Model file for the job. Use its own axes, mm. A direction names the side the tool comes from. Round coordinates to 2 decimals unless told otherwise and drop trailing zeros. Order: outer loops, then holes, each group sorted by start corner. A loop starts at its lowest first (then second) coordinate and runs counter-clockwise, first axis right, second up. Notation, with made-up numbers: (55, 35.25) - (89, 35.25) arc R21 cw to (89, 60.25) - close; hole circle Ø6 at (-9.5, 73). An arc over 180 degrees is marked (long way). Write item = value, one per line. Start each with the question number.
Autodesk Inventor part; units mm, degrees
ref_plane "YZ Plane" through (0, 0, 0) normal (1, 0, 0) x (0, 1, 0)
ref_plane "XZ Plane" through (0, 0, 0) normal (0, 1, 0) x (-1, 0, 0)
ref_plane "XY Plane" through (0, 0, 0) normal (0, 0, 1) x (1, 0, 0)
sketch "Sketch1" plane through (0, 0, 0) normal (0, 0, 1) x (1, 0, 0)
  line L0 (-9.652, -11.176) -> (9.652, -11.176)
  arc A0 (-11.176, -9.652) -> (-9.652, -11.176) centre (-9.652, -9.652) ccw
  line L1 (-11.176, 9.652) -> (-11.176, -9.652)
  arc A1 (-9.652, 11.176) -> (-11.176, 9.652) centre (-9.652, 9.652) ccw
  line L2 (9.652, 11.176) -> (-9.652, 11.176)
  arc A2 (11.176, 9.652) -> (9.652, 11.176) centre (9.652, 9.652) ccw
  line L3 (11.176, -9.652) -> (11.176, 9.652)
  arc A3 (9.652, -11.176) -> (11.176, -9.652) centre (9.652, -9.652) ccw
  arc A4 (12.7, 6.731) -> (13.081, 6.35) centre (13.081, 6.731) ccw
  line L4 (12.7, 6.731) -> (12.7, 10.5918)
  arc A5 (12.7, 10.5918) -> (10.5918, 12.7) centre (10.5918, 10.5918) ccw
  line L5 (10.5918, 12.7) -> (-10.5918, 12.7)
  arc A6 (-10.5918, 12.7) -> (-12.7, 10.5918) centre (-10.5918, 10.5918) ccw
  line L6 (-12.7, 10.5918) -> (-12.7, 6.731)
  arc A7 (-13.081, 6.35) -> (-12.7, 6.731) centre (-13.081, 6.731) ccw
  line L7 (-13.081, 6.35) -> (-25.019, 6.35)
  arc A8 (-25.019, 6.35) -> (-25.4, 5.969) centre (-25.019, 5.969) ccw
  line L8 (-25.4, 5.969) -> (-25.4, 4.826)
  arc A9 (-25.4, 4.826) -> (-24.638, 4.064) centre (-24.638, 4.826) ccw
  line L9 (-24.638, 4.064) -> (-23.0632, 4.064)
  arc A10 (-23.0632, 4.064) -> (-22.6822, 4.445) centre (-23.0632, 4.445) ccw
  arc A11 (-22.3012, 4.826) -> (-22.6822, 4.445) centre (-22.3012, 4.445) ccw
  line L10 (-22.3012, 4.826) -> (-13.081, 4.826)
  arc A12 (-12.7, 4.445) -> (-13.081, 4.826) centre (-13.081, 4.445) ccw
  line L11 (-12.7, 4.445) -> (-12.7, -4.445)
  arc A13 (-13.081, -4.826) -> (-12.7, -4.445) centre (-13.081, -4.445) ccw
  line L12 (-13.081, -4.826) -> (-22.3012, -4.826)
  arc A14 (-22.6822, -4.445) -> (-22.3012, -4.826) centre (-22.3012, -4.445) ccw
  arc A15 (-22.6822, -4.445) -> (-23.0632, -4.064) centre (-23.0632, -4.445) ccw
  line L13 (-23.0632, -4.064) -> (-24.638, -4.064)
  arc A16 (-24.638, -4.064) -> (-25.4, -4.826) centre (-24.638, -4.826) ccw
  line L14 (-25.4, -4.826) -> (-25.4, -5.969)
  arc A17 (-25.4, -5.969) -> (-25.019, -6.35) centre (-25.019, -5.969) ccw
  line L15 (-25.019, -6.35) -> (-13.081, -6.35)
  arc A18 (-12.7, -6.731) -> (-13.081, -6.35) centre (-13.081, -6.731) ccw
  line L16 (-12.7, -6.731) -> (-12.7, -10.5918)
  arc A19 (-12.7, -10.5918) -> (-10.5918, -12.7) centre (-10.5918, -10.5918) ccw
  line L17 (-10.5918, -12.7) -> (10.5918, -12.7)
  arc A20 (10.5918, -12.7) -> (12.7, -10.5918) centre (10.5918, -10.5918) ccw
  line L18 (12.7, -10.5918) -> (12.7, -6.731)
  arc A21 (13.081, -6.35) -> (12.7, -6.731) centre (13.081, -6.731) ccw
  line L19 (13.081, -6.35) -> (25.019, -6.35)
  arc A22 (25.019, -6.35) -> (25.4, -5.969) centre (25.019, -5.969) ccw
  line L20 (25.4, -5.969) -> (25.4, -4.826)
  arc A23 (25.4, -4.826) -> (24.638, -4.064) centre (24.638, -4.826) ccw
  line L21 (24.638, -4.064) -> (23.0632, -4.064)
  arc A24 (23.0632, -4.064) -> (22.6822, -4.445) centre (23.0632, -4.445) ccw
  arc A25 (22.3012, -4.826) -> (22.6822, -4.445) centre (22.3012, -4.445) ccw
  line L22 (22.3012, -4.826) -> (13.081, -4.826)
  arc A26 (12.7, -4.445) -> (13.081, -4.826) centre (13.081, -4.445) ccw
  line L23 (12.7, -4.445) -> (12.7, 4.445)
  arc A27 (13.081, 4.826) -> (12.7, 4.445) centre (13.081, 4.445) ccw
  line L24 (13.081, 4.826) -> (22.3012, 4.826)
  arc A28 (22.6822, 4.445) -> (22.3012, 4.826) centre (22.3012, 4.445) ccw
  arc A29 (22.6822, 4.445) -> (23.0632, 4.064) centre (23.0632, 4.445) ccw
  line L25 (23.0632, 4.064) -> (24.638, 4.064)
  arc A30 (24.638, 4.064) -> (25.4, 4.826) centre (24.638, 4.826) ccw
  line L26 (25.4, 4.826) -> (25.4, 5.969)
  arc A31 (25.4, 5.969) -> (25.019, 6.35) centre (25.019, 5.969) ccw
  line L27 (25.019, 6.35) -> (13.081, 6.35)
  point P0 (0, 0)
extrude "Extrusion1" add sketch "Sketch1" against normal blind 304.8
properties part number "9035"
Item 1: Mould opens along X. For faces 1 (the face through (-11.176, 0, -150)), 2 (the face through (19, -6.35, -150)) say: +X half, -X half, draft (parallel to the pull), parting line (faces both ways), or undercut.
Item 2: Saw through at A-A, the plane x = -18. Give the cut face in (y, z).
Item 3: Drop flat-ended pins along their axis: pin 1 (3 mm diameter, centred on y = -9, z = -213.5, fed in from -X); pin 2 (10 mm diameter, centred on x = -19, z = -87.5, fed in from +Y); pin 3 (1.3 mm diameter, centred on x = 24, z = -118.5, fed in from -Y). Give the stop position or say it passes through.
Item 4: Probe L1, parallel to X at y = 7, z = -275; L2, parallel to Y at x = -18, z = -76.5. List the from-to ranges inside material, lowest first.
Item 5: Which spindle directions (+Z, -Z, +X, -X, +Y, -Y) get a long thin tool onto all of the face, cutting with end or side? Do faces 3 (the face through (0, -12.7, -150)), 4 (the face through (-18, 4.826, -150)), 5 (the face through (-19, -6.35, -150)), 6 (the face through (19, 6.35, -150)), 7 (the face through (-19, 6.35, -150)). Say none if no direction does.
Check sheet entries:
q1.face_1 = undercut
q1.face_2 = draft
q2.outline = (-6.35, -304.8) - (-4.83, -304.8) - (-4.83, 0) - (-6.35, 0) - close; (4.83, -304.8) - (6.35, -304.8) - (6.35, 0) - (4.83, 0) - close
q3.pin_1 = -12.7
q3.pin_2 = 6.35
q3.pin_3 = -6.35
q4.L1 = -12.7 to -11.18, 11.18 to 12.7
q4.L2 = -6.35 to -4.83, 4.83 to 6.35
q5.face_3 = +Z, -Z, +X, -X, -Y
q5.face_4 = +Z, -Z
q5.face_5 = +Z, -Z, -X, -Y
q5.face_6 = +Z, -Z, +X, +Y
q5.face_7 = +Z, -Z, -X, +Y
